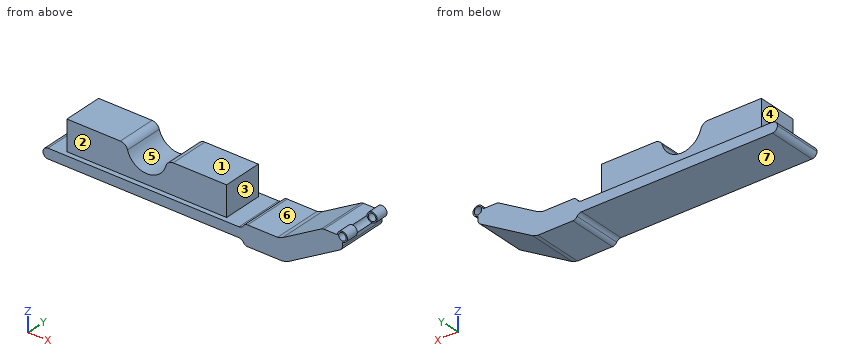
```python
from build123d import *

# Parameters (mm, degrees)
F1_DEPTH      = 31.75
F1_DEPTH_BACK = 31.75
F2_DEPTH      = 25.4
F2_DEPTH_BACK = 25.4
F4_R          = 6.35
F5_DEPTH      = 31.75


with BuildPart() as f1:
    # F0 (on Front) → F1 (new body, two sides)
    with BuildSketch(Plane.XZ) as f1_sk:
        with BuildLine():
            Line((0, -11.0555849444), (0, -6.35))
            ThreePointArc((0, -6.35), (4.4901280605, 4.4901280605), (-6.35, 0))
            Line((-6.35, 0), (-23.488145619, 0))
            ThreePointArc((-23.488145619, 0), (-25.145368487, -0.2200642446), (-26.6877266311, -0.8650039793))
            Line((-26.6877266311, -0.8650039793), (-76.2, -29.7471634445))
            Line((-76.2, -29.7471634445), (-82.5991620242, -31.75))
            Line((-82.5991620242, -31.75), (-120.65, -31.75))
            ThreePointArc((-120.65, -31.75), (-123.825, -32.600738686), (-126.149261314, -34.925))
            ThreePointArc((-126.149261314, -34.925), (-128.4735226281, -37.249261314), (-131.6485226281, -38.1))
            Line((-131.6485226281, -38.1), (-152.4, -38.1))
            Line((-152.4, -38.1), (-355.6, -38.1))
            Line((-355.6, -38.1), (-374.65, -38.1))
            ThreePointArc((-374.65, -38.1), (-379.1401280605, -39.9598719395), (-381, -44.45))
            ThreePointArc((-381, -44.45), (-379.1401280605, -48.9401280605), (-374.65, -50.8))
            Line((-374.65, -50.8), (-131.6485226281, -50.8))
            ThreePointArc((-131.6485226281, -50.8), (-128.4735226281, -51.650738686), (-126.149261314, -53.975))
            ThreePointArc((-126.149261314, -53.975), (-123.825, -56.299261314), (-120.65, -57.15))
            Line((-120.65, -57.15), (-76.2, -57.15))
            Line((-76.2, -57.15), (-69.8008379758, -55.4199920414))
            Line((-69.8008379758, -55.4199920414), (-3.1504189879, -16.5405809651))
            ThreePointArc((-3.1504189879, -16.5405809651), (-0.8436473312, -14.2182705574), (0, -11.0555849444))
        make_face()
        with BuildLine():
            ThreePointArc((-4.7625, 0), (0, 4.7625), (4.7625, 0))
            ThreePointArc((4.7625, 0), (0, -4.7625), (-4.7625, 0))
        make_face(mode=Mode.SUBTRACT)
    extrude(amount=F1_DEPTH)
    extrude(f1_sk.sketch, amount=-F1_DEPTH_BACK)

    # F0 (on Front) → F2 (join, two sides)
    with BuildSketch(Plane.XZ) as f2_sk:
        with BuildLine():
            Line((0, -11.0555849444), (0, -6.35))
            ThreePointArc((0, -6.35), (4.4901280605, 4.4901280605), (-6.35, 0))
            Line((-6.35, 0), (-23.488145619, 0))
            ThreePointArc((-23.488145619, 0), (-25.145368487, -0.2200642446), (-26.6877266311, -0.8650039793))
            Line((-26.6877266311, -0.8650039793), (-76.2, -29.7471634445))
            Line((-76.2, -29.7471634445), (-82.5991620242, -31.75))
            Line((-82.5991620242, -31.75), (-120.65, -31.75))
            ThreePointArc((-120.65, -31.75), (-123.825, -32.600738686), (-126.149261314, -34.925))
            ThreePointArc((-126.149261314, -34.925), (-128.4735226281, -37.249261314), (-131.6485226281, -38.1))
            Line((-131.6485226281, -38.1), (-152.4, -38.1))
            Line((-152.4, -38.1), (-355.6, -38.1))
            Line((-355.6, -38.1), (-374.65, -38.1))
            ThreePointArc((-374.65, -38.1), (-379.1401280605, -39.9598719395), (-381, -44.45))
            ThreePointArc((-381, -44.45), (-379.1401280605, -48.9401280605), (-374.65, -50.8))
            Line((-374.65, -50.8), (-131.6485226281, -50.8))
            ThreePointArc((-131.6485226281, -50.8), (-128.4735226281, -51.650738686), (-126.149261314, -53.975))
            ThreePointArc((-126.149261314, -53.975), (-123.825, -56.299261314), (-120.65, -57.15))
            Line((-120.65, -57.15), (-76.2, -57.15))
            Line((-76.2, -57.15), (-69.8008379758, -55.4199920414))
            Line((-69.8008379758, -55.4199920414), (-3.1504189879, -16.5405809651))
            ThreePointArc((-3.1504189879, -16.5405809651), (-0.8436473312, -14.2182705574), (0, -11.0555849444))
        make_face()
        with BuildLine():
            ThreePointArc((-4.7625, 0), (0, 4.7625), (4.7625, 0))
            ThreePointArc((4.7625, 0), (0, -4.7625), (-4.7625, 0))
        make_face(mode=Mode.SUBTRACT)
        with BuildLine():
            Line((-355.6, -38.1), (-152.4, -38.1))
            Line((-152.4, -38.1), (-152.4, 0))
            Line((-152.4, 0), (-220.3989583495, 0))
            ThreePointArc((-220.3989583495, 0), (-226.1427494637, -1.9266785646), (-229.5628787996, -6.9272727273))
            ThreePointArc((-229.5628787996, -6.9272727273), (-254, -25.4), (-278.4371212004, -6.9272727273))
            ThreePointArc((-278.4371212004, -6.9272727273), (-281.8572505363, -1.9266785646), (-287.6010416505, 0))
            Line((-287.6010416505, 0), (-355.6, 0))
            Line((-355.6, 0), (-355.6, -38.1))
        make_face()
    extrude(amount=F2_DEPTH)
    extrude(f2_sk.sketch, amount=-F2_DEPTH_BACK)

    # F4 (on offset) → F5 (cut)
    with BuildSketch(Plane.XZ.offset(15.875)):
        Circle(F4_R)
    extrude(amount=-F5_DEPTH, mode=Mode.SUBTRACT)


solid = f1.part
```
Build history of the part. All positions in model axes, mm. Face numbers are marked on the shaded views. A direction names the side the tool comes from. Coordinates: 2 decimals unless noted, no trailing zeros. Order: outer loops, then holes, each group sorted by start corner. A loop starts at its lowest first (then second) coordinate and runs counter-clockwise, first axis right, second up. Notation, with made-up numbers: (18, 12.5) -> (72, 12.5) arc R36 ccw to (72, 47.5) -> close; hole circle Ø10 at (-39.75, 3.25). An arc over 180 degrees is marked (long way). Answer in a Markdown table with one row per item. Add a question column.
Q1. Drop flat-ended pins along their axis: pin 1 (1.5 mm diameter, centred on y = -13.5, z = -7, fed in from +X); pin 2 (1 mm diameter, centred on x = -61.5, y = 22, fed in from +Z); pin 3 (11.5 mm diameter, centred on x = -302.5, z = -9.5, fed in from +Y). Give the stop position or say it passes through.
Q2. Mould opens along X. For the marked faces 4, 5, 6 and 7 say: +X half, -X half, draft (parallel to the pull), parting line (faces both ways), or undercut.
Q3. Band-saw the part on D-D, the plane x = -47.5. List the corners of the cut face in (y, z).
Q4. Wall check: line 1 along X through (y, z) = (-19.5, -3); line 2 along X through (y, z) = (10, -8); line 3 along X through (y, z) = (-23.5, -3.5). Give the ranges that are in metal, low to high. Write a range as [from, to].
Q5. Band-saw the part on B-B, the plane y = -2. List the corners of the cut face in (x, z) (3 decimals).
Q6. Band-saw the part on C-C, the plane x = -116. List the corners of the cut face in (y, z).
Q7. Which spindle directions (+Z, -Z, +X, -X, +Y, -Y) get a long thin tool onto all of the face, cutting with end or side? Do the marked faces 1, 2 and 3. Say none if no direction does.
Q8. Band-saw the part on A-A, the plane x = -351.5. List the corners of the cut face in (y, z).
Answers follow:
| question | item | result |
|---|---|---|
| 1 | pin 1 | x = 0 |
| 1 | pin 2 | z = -20.88 |
| 1 | pin 3 | y = 25.4 |
| 2 | face 4 | -X half |
| 2 | face 5 | undercut |
| 2 | face 6 | undercut |
| 2 | face 7 | draft |
| 3 | outline | (-31.75, -42.41) -> (31.75, -42.41) -> (31.75, -13.01) -> (-31.75, -13.01) -> close |
| 4 | line 1 | [-355.6, -280.66], [-227.34, -152.4], [-30.35, -3.7], [3.7, 5.6] |
| 4 | line 2 | [-355.6, -278.11], [-229.89, -152.4], [-38.92, 0] |
| 4 | line 3 | [-355.6, -280.22], [-227.78, -152.4], [-31.2, -3.23], [3.23, 5.3] |
| 5 | outline | (-374.65, -50.8) -> (-131.649, -50.8) arc R6.35 cw to (-126.149, -53.975) arc R6.35 ccw to (-120.65, -57.15) -> (-76.2, -57.15) -> (-69.801, -55.42) -> (-3.15, -16.541) arc R6.35 ccw to (0, -11.056) -> (0, -6.35) arc R6.35 cw to (-6.35, 0) -> (-23.488, 0) arc R6.35 ccw to (-26.688, -0.865) -> (-76.2, -29.747) -> (-82.599, -31.75) -> (-120.65, -31.75) arc R6.35 ccw to (-126.149, -34.925) arc R6.35 cw to (-131.649, -38.1) -> (-152.4, -38.1) -> (-152.4, 0) -> (-220.399, 0) arc R9.525 ccw to (-229.563, -6.927) arc R25.4 cw to (-278.437, -6.927) arc R9.525 ccw to (-287.601, 0) -> (-355.6, 0) -> (-355.6, -38.1) -> (-374.65, -38.1) arc R6.35 ccw to start |
| 6 | outline | (-31.75, -57.15) -> (31.75, -57.15) -> (31.75, -31.75) -> (-31.75, -31.75) -> close |
| 7 | face 1 | +Z, -X, +Y, -Y |
| 7 | face 2 | +Z, -X, -Y |
| 7 | face 3 | +Z, +Y, -Y |
| 8 | outline | (-31.75, -50.8) -> (31.75, -50.8) -> (31.75, -38.1) -> (25.4, -38.1) -> (25.4, 0) -> (-25.4, 0) -> (-25.4, -38.1) -> (-31.75, -38.1) -> close |
